Autodesk Inventor part; units mm, degrees
ref_plane "Начальная плоскость" through (0, 0, -10) normal (0, 0, 1) x (1, 0, 0)
ref_plane "Конечная плоскость" through (0, 0, 340) normal (0, 0, 1) x (1, 0, 0)
ref_plane "РабПлоскость4" through (-600, 0, -10) normal (0, 0, -1) x (-1, 0, 0)
ref_plane "Начальная плоскость" through (0, 0, -10) normal (0, 0, 1) x (1, 0, 0)
ref_plane "Конечная плоскость" through (0, 0, 340) normal (0, 0, 1) x (1, 0, 0)
sketch "Эскиз" plane through (0, 0, 0) normal (0, 0, 1) x (1, 0, 0)
  line L0 (-14.4349, 0) -> (14.4349, 0)
  line L1 (0, -14) -> (0, 14)
  line L2 (0, 0) -> (7.5, 7.5) construction
  circle A0 centre (7.5, 7.5) radius 1.65 construction
  line L3 (5.85, 9.15) -> (9.15, 9.15)
  line L4 (9.15, 9.15) -> (9.15, 5.85)
  line L5 (9.15, 5.85) -> (5.85, 5.85)
  line L6 (5.85, 5.85) -> (5.85, 9.15)
  line L7 (3.235, 8.1636) -> (4.72, 9.9636)
  line L8 (4.7971, 10) -> (8.5, 10)
  line L9 (3.3121, 8) -> (4.95, 8)
  line L10 (4.95, 8) -> (4.95, 5.7985)
  line L11 (4.95, 5.7985) -> (2.6515, 3.5)
  line L12 (0, 3.5) -> (2.6515, 3.5)
  circle A1 centre (0, 0) radius 2.5
  line L13 (8.1636, 3.235) -> (9.9636, 4.72)
  line L14 (10, 4.7971) -> (10, 8.5)
  line L15 (8, 3.3121) -> (8, 4.95)
  line L16 (8, 4.95) -> (5.7985, 4.95)
  line L17 (5.7985, 4.95) -> (3.5, 2.6515)
  line L18 (3.5, 0) -> (3.5, 2.6515)
  arc A2 (10, 8.5) -> (8.5, 10) centre (8.5, 8.5) ccw
  line L19 (0, 0) -> (-7.5, 7.5) construction
  circle A3 centre (-7.5, 7.5) radius 1.65 construction
  line L20 (-5.85, 9.15) -> (-9.15, 9.15)
  line L21 (-9.15, 9.15) -> (-9.15, 5.85)
  line L22 (-9.15, 5.85) -> (-5.85, 5.85)
  line L23 (-5.85, 5.85) -> (-5.85, 9.15)
  line L24 (-3.235, 8.1636) -> (-4.72, 9.9636)
  line L25 (-4.7971, 10) -> (-8.5, 10)
  line L26 (-3.3121, 8) -> (-4.95, 8)
  line L27 (-4.95, 8) -> (-4.95, 5.7985)
  line L28 (-4.95, 5.7985) -> (-2.6515, 3.5)
  line L29 (0, 3.5) -> (-2.6515, 3.5)
  line L30 (-3.5, 0) -> (-3.5, 2.6515)
  line L31 (-5.7985, 4.95) -> (-3.5, 2.6515)
  line L32 (-8, 4.95) -> (-5.7985, 4.95)
  line L33 (-8, 3.3121) -> (-8, 4.95)
  line L34 (-8.1636, 3.235) -> (-9.9636, 4.72)
  line L35 (-10, 4.7971) -> (-10, 8.5)
  arc A4 (-8.5, 10) -> (-10, 8.5) centre (-8.5, 8.5) ccw
  line L36 (0, 14) -> (0, -14)
  line L37 (0, 0) -> (7.5, -7.5) construction
  circle A5 centre (7.5, -7.5) radius 1.65 construction
  line L38 (5.85, -9.15) -> (9.15, -9.15)
  line L39 (9.15, -9.15) -> (9.15, -5.85)
  line L40 (9.15, -5.85) -> (5.85, -5.85)
  line L41 (5.85, -5.85) -> (5.85, -9.15)
  line L42 (3.235, -8.1636) -> (4.72, -9.9636)
  line L43 (4.7971, -10) -> (8.5, -10)
  line L44 (3.3121, -8) -> (4.95, -8)
  line L45 (4.95, -8) -> (4.95, -5.7985)
  line L46 (4.95, -5.7985) -> (2.6515, -3.5)
  line L47 (0, -3.5) -> (2.6515, -3.5)
  line L48 (3.5, 0) -> (3.5, -2.6515)
  line L49 (5.7985, -4.95) -> (3.5, -2.6515)
  line L50 (8, -4.95) -> (5.7985, -4.95)
  line L51 (8, -3.3121) -> (8, -4.95)
  line L52 (8.1636, -3.235) -> (9.9636, -4.72)
  line L53 (10, -4.7971) -> (10, -8.5)
  arc A6 (8.5, -10) -> (10, -8.5) centre (8.5, -8.5) ccw
  line L54 (0, 0) -> (-7.5, -7.5) construction
  line L55 (-4.95, -8) -> (-4.95, -5.7985)
  line L56 (-3.3121, -8) -> (-4.95, -8)
  line L57 (-5.7985, -4.95) -> (-3.5, -2.6515)
  line L58 (-4.95, -5.7985) -> (-2.6515, -3.5)
  line L59 (-3.5, 0) -> (-3.5, -2.6515)
  line L60 (0, -3.5) -> (-2.6515, -3.5)
  circle A7 centre (-7.5, -7.5) radius 1.65 construction
  line L61 (-5.85, -5.85) -> (-5.85, -9.15)
  line L62 (-5.85, -9.15) -> (-9.15, -9.15)
  line L63 (-9.15, -9.15) -> (-9.15, -5.85)
  line L64 (-9.15, -5.85) -> (-5.85, -5.85)
  line L65 (-3.235, -8.1636) -> (-4.72, -9.9636)
  line L66 (-8, -4.95) -> (-5.7985, -4.95)
  line L67 (-8, -3.3121) -> (-8, -4.95)
  line L68 (-8.1636, -3.235) -> (-9.9636, -4.72)
  line L69 (-4.7971, -10) -> (-8.5, -10)
  line L70 (-10, -4.7971) -> (-10, -8.5)
  arc A8 (-10, -8.5) -> (-8.5, -10) centre (-8.5, -8.5) ccw
  arc A9 (3.235, 8.1636) -> (3.3121, 8) centre (3.3121, 8.1) ccw
  arc A10 (4.7971, 10) -> (4.72, 9.9636) centre (4.7971, 9.9) ccw
  arc A11 (8, 3.3121) -> (8.1636, 3.235) centre (8.1, 3.3121) ccw
  arc A12 (9.9636, 4.72) -> (10, 4.7971) centre (9.9, 4.7971) ccw
  arc A13 (-3.3121, 8) -> (-3.235, 8.1636) centre (-3.3121, 8.1) ccw
  arc A14 (-4.72, 9.9636) -> (-4.7971, 10) centre (-4.7971, 9.9) ccw
  arc A15 (-8.1636, 3.235) -> (-8, 3.3121) centre (-8.1, 3.3121) ccw
  arc A16 (-10, 4.7971) -> (-9.9636, 4.72) centre (-9.9, 4.7971) ccw
  arc A17 (-8, -3.3121) -> (-8.1636, -3.235) centre (-8.1, -3.3121) ccw
  arc A18 (-9.9636, -4.72) -> (-10, -4.7971) centre (-9.9, -4.7971) ccw
  arc A19 (-3.235, -8.1636) -> (-3.3121, -8) centre (-3.3121, -8.1) ccw
  arc A20 (-4.7971, -10) -> (-4.72, -9.9636) centre (-4.7971, -9.9) ccw
  arc A21 (4.72, -9.9636) -> (4.7971, -10) centre (4.7971, -9.9) ccw
  arc A22 (3.3121, -8) -> (3.235, -8.1636) centre (3.3121, -8.1) ccw
  arc A23 (8.1636, -3.235) -> (8, -3.3121) centre (8.1, -3.3121) ccw
  arc A24 (10, -4.7971) -> (9.9636, -4.72) centre (9.9, -4.7971) ccw
  point P0 (3.1, 8)
  point P1 (4.75, 10)
  point P2 (7.5, 9.15)
  point P3 (8, 3.1)
  point P4 (10, 4.75)
  point P5 (7.5, 5.85)
  point P6 (9.15, 7.5)
  point P7 (-3.1, 8)
  point P8 (-4.75, 10)
  point P9 (-7.5, 9.15)
  point P10 (-8, 3.1)
  point P11 (-10, 4.75)
  point P12 (-7.5, 5.85)
  point P13 (-9.15, 7.5)
  point P14 (3.1, -8)
  point P15 (4.75, -10)
  point P16 (7.5, -9.15)
  point P17 (8, -3.1)
  point P18 (10, -4.75)
  point P19 (7.5, -5.85)
  point P20 (9.15, -7.5)
  point P21 (-3.1, -8)
  point P22 (-7.5, -5.85)
  point P23 (-7.5, -9.15)
  point P24 (-9.15, -7.5)
  point P25 (-4.75, -10)
  point P26 (-8, -3.1)
  point P27 (-10, -4.75)
  dimension "d0" = 45
  dimension "d1" = 3.3
  dimension "d2" = 1.5
  dimension "d3" = 1.2
  dimension "d4" = 5
  dimension "d5" = 6.5
  dimension "d6" = 15
  dimension "d7" = 20
  dimension "d8" = 9.9
  dimension "d9" = 9.5
  dimension "d10" = 6.2
  dimension "d11" = 2
  dimension "d18" = 0.1
  dimension "d19" = 0.1
extrude "Тело" add sketch "Эскиз" along normal up to surface (350 mm away) from surface at -10 contours A1 L1 L12 L11 L10 L9 A9 L7 A10 L8 A2 L14 A12 L13 A11 L15 L16 L17 L18 L0 | L0 L48 L49 L50 L51 A23 L52 A24 L53 A6 L43 A21 L42 A22 L44 L45 L46 L47 L1 A1 | A1 L0 L30 L31 L32 L33 A15 L34 A16 L35 A4 L25 A14 L24 A13 L26 L27 L28 L29 L1 | L1 L60 L58 L55 L56 A19 L65 A20 L69 A8 L70 A18 L68 A17 L67 L66 L57 L59 L0 A1
sketch "Эскиз2" plane through (0, 0, 0) normal (0, 0, 1) x (1, 0, 0)
  line L0 (0, 0) -> (10, 0)
ref_plane "РабПлоскость3" through (0, 0, 0) normal (0, -1, 0) x (1, 0, 0)
sketch "Эскиз3" plane through (0, 0, 0) normal (0, -1, 0) x (1, 0, 0)
  line L0 (-2, -10) -> (12, -10)
  line L1 (-2, 340) -> (12, 340)
  dimension "d25" = 350
ref_plane "РабПлоскость4" through (-600, 0, -10) normal (0, 0, -1) x (-1, 0, 0)
split "Разделение1" plane through (-600, 0, -10) removes the side toward (0, 0, -1)
ref_plane "РабПлоскость5" through (0, 0, -10) normal (0, 0, -1) x (-1, 0, 0)
split "Разделение2" plane through (0, 0, -10) removes the side toward (0, 0, -1)
ref_plane "РабПлоскость6" through (-500, 0, 340) normal (0, 0, 1) x (1, 0, 0)
split "Разделение3" plane through (-500, 0, 340) removes the side toward (0, 0, 1)
ref_plane "РабПлоскость7" through (0, 10, 340) normal (0, 0, 1) x (1, 0, 0)
split "Разделение4" plane through (0, 10, 340) removes the side toward (0, 0, 1)
properties part number "короткая палка" material "Алюминий 6061"
Geometry: final body of the model. Coordinates: model frame, mm. A direction names the side the tool comes from. Give positions to 0.01 mm unless a question says otherwise; leave off trailing zeros. Return JSON: item names as keys, results as strings.
Item 1: Line query: line 1 (Y direction, x = 6.75, z = 189.5); line 2 (X direction, y = 0, z = 79). Output: solid intervals per line, ascending.
Filled in:
{"line 1": "-10 to -9.15, -5.85 to -4.95, 4.95 to 5.85, 9.15 to 10", "line 2": "-3.5 to -2.5, 2.5 to 3.5"}
Item 2: Access query for faces 1 (the flat face through (0, -3.5, 163)), 2 (the flat face through (0, 3.5, 163)), 3 (the flat face through (3.5, 0, 163)), 4 (the flat face through (-3.5, 0, 163)). Directions: +Z, -Z, +X, -X, +Y, -Y. A direction counts if a zero-diameter tool reaches every point of the face in a straight line with its end or side. Return the directions, or none.
Filled in:
{"face 1": "+Z, -Z, -Y", "face 2": "+Z, -Z, +Y", "face 3": "+Z, -Z, +X", "face 4": "+Z, -Z, -X"}
Item 3: Pin query (flat end, axial travel): P1, Ø2.5, axis at x = -1, z = 172.5, coming from the +Y side; P2, Ø1.3, axis at x = 3.5, z = 124.5, coming from the +Y side; P3, Ø1.3, axis at y = -4, z = 108.5, coming from the +X side. Return the tip coordinate at first contact, or that it passes through.
Filled in:
{"P1": "y = 3.5", "P2": "y = 9.27", "P3": "x = 9.88"}
Item 4: Section A-A, the plane z = 286. Count the separate pieces of the cut face and the enclosed holes in it, plus the area to 3 significant figures.
Filled in:
{"separate pieces": "1", "enclosed holes": "5", "area": "115 mm^2"}
